Check sheet for the modelled part. Datum: model origin and axes. Units: mm. A direction names the side the tool comes from. Coordinates: 2 decimals unless noted, no trailing zeros. Loops run counter-clockwise (first coordinate to the right, second up) from the corner with the lowest first, then second, coordinate; pieces in that order, holes last. Notation, with made-up numbers: (4, 38) - (34, 38) arc R22 ccw to (34, 56) - close; hole circle Ø6 at (-16, -26). An arc over 180 degrees is marked (long way). Write each question's results on one line, items separated by ' | '. Start each with the question number.
1. Cross-section at D-D (y = 52). Record the cut outline in (x, z).
2. Cross-section at A-A (y = 7). Record the cut outline in (x, z).
3. Tool access check on faces 4 (the face through (35.56, -1, 10)), 5 (the face through (37, -38.1, 10)). Record the directions out of +Z, -Z, +X, -X, +Y, -Y that give a thin tool (end or side, any length) a straight path to the whole face; none if there is none.
4. Thickness scan on line 1 (X direction, y = 4.5, z = 16); line 2 (X direction, y = 41, z = 6.25); line 3 (Y direction, x = -2, z = 7). Record the ranges inside material, lowest first. Write a range as [from, to].
5. Draft check along X on faces 1 (the face through (38.1, -1, 10)), 2 (the face through (-35.56, -1, 10)), 3 (the face through (37, 28, 20.32)). Enter one of: released by +X, released by -X, zero draft, split by the parting line, or undercut.
6. Cross-section at C-C (x = 0). Record the cut outline in (y, z), and give its area (3 significant figures).
7. Cross-section at B-B (z = 16). Record the cut outline in (x, y), and give its area (3 significant figures).
8. Gauge pin test, flat ends, axial feed: P1, Ø6, axis at x = -1.5, z = 18.5, coming from the +Y side; P2, Ø4, axis at x = 16.5, z = 7.5, coming from the +Y side; P3, Ø2, axis at x = -6.5, z = 3.5, coming from the +Y side; P4, Ø10, axis at x = -26.5, y = 32, coming from the -Z side. Record the tip position at first contact, or that the pin passes through.
```python
from build123d import *

# Parameters (mm, degrees)
F0_W     = 76.2
F0_H     = 76.2
F1_DEPTH = 20.066
F2_DEPTH = 0.254
F3_T     = -2.54


with BuildPart() as f1:
    # F0 (on Top) → F1 (new body)
    with BuildSketch(Plane.XY):
        Rectangle(F0_W, F0_H)
        with BuildLine():
            Line((-38.1, 38.1), (38.1, 38.1))
            ThreePointArc((38.1, 38.1), (0, 76.2), (-38.1, 38.1))
        make_face()
    extrude(amount=F1_DEPTH)

    # F2 (add): a face of the model
    f2_faces = [f1.faces().sort_by_distance(p)[0] for p in [
        (0, 15.3025411539, 20.066),
    ]]
    extrude(f2_faces, amount=F2_DEPTH)

    # F3
    f3_openings = [f1.faces().sort_by_distance(p)[0] for p in [
        (0, -38.1, 10.16),
        (0, 15.302541, 20.32),
        (0, 15.302541, 0),
    ]]
    offset(amount=F3_T, openings=f3_openings)


solid = f1.part
```
Established:
1) outline: (-35.47, 0) - (-32.73, 0) - (-32.73, 20.32) - (-35.47, 20.32) - close; (32.73, 0) - (35.47, 0) - (35.47, 20.32) - (32.73, 20.32) - close
2) outline: (-38.1, 0) - (-35.56, 0) - (-35.56, 20.32) - (-38.1, 20.32) - close; (35.56, 0) - (38.1, 0) - (38.1, 20.32) - (35.56, 20.32) - close
3) face 4: +Z, -Z, -Y | face 5: +Z, -Z, +X, -X, -Y
4) line 1: [-38.1, -35.56], [35.56, 38.1] | line 2: [-37.99, -35.44], [35.44, 37.99] | line 3: [73.6, 76.15]
5) face 1: released by +X | face 2: undercut | face 3: zero draft
6) outline: (73.66, 0) - (76.2, 0) - (76.2, 20.32) - (73.66, 20.32) - close | area: 51.6 mm^2
7) outline: (-38.1, -38.1) - (-35.56, -38.1) - (-35.56, 38.1) arc R35.56 cw to (35.56, 38.1) - (35.56, -38.1) - (38.1, -38.1) - (38.1, 38.1) arc R38.1 ccw to (-38.1, 38.1) - close | area: 681 mm^2
8) P1: y = 76.2 | P2: y = 73.33 | P3: y = 75.8 | P4: through
